Read the model definition and answer for the solid it produces. Units are mm, in the model's axes. Face numbers are marked on the shaded views. A direction names the side the tool comes from. Give positions to 0.01 mm unless a question says otherwise; leave off trailing zeros. Order: outer loops, then holes, each group sorted by start corner. A loop starts at its lowest first (then second) coordinate and runs counter-clockwise, first axis right, second up.
Item 1: Find the intervals of material crossed by line 1 along Y through (x, z) = (-18, 0.9); line 2 along X through (y, z) = (-19.5, 5.5); line 3 along X through (y, z) = (26, 0.55), in increasing order.
Item 2: A cutting plane is placed at D-D (z = 1.9). State how many separate pieces and enclosed holes the cut face has, plus the area to 3 significant figures.
Item 3: Which of the six approach directions +Z, -Z, +X, -X, +Y, -Y give full straight-line access (tool end or side, diameter ignored) to the marked faces 1, 2 and 3?
Item 4: A cutting plane is placed at A-A (y = 21). Write down the section's boundary in (x, z), plus the area to 3 significant figures.
Item 5: Given pin 1 Ø2 at (x, y) = (-4.5, 7) entering from +Z; pin 2 Ø2 at (y, z) = (19.5, 2) entering from +X; pin 3 Ø5 at (x, y) = (7, 24) entering from +Z (3 decimals), each flat-ended and moving along its own axis, determine where each tip first touches the part or whether it passes through.
Item 6: A cutting plane is placed at C-C (x = -5). Write down the section's boundary in (y, z).
Item 7: A cutting plane is placed at B-B (y = 4.5). Write down the section's boundary in (x, z), plus the area to 3 significant figures.
Item 8: The mould has two halves that part along X. Classify the marked faces 4, 5 and 6: +X half, -X half, draft (parallel to the pull), parting line (faces both ways), or undercut.
Autodesk Fusion 360 part; units mm, degrees
sketch "Sketch1" plane through (0, 0, 0) normal (0, 0, 1) x (1, 0, 0)
  circle A0 centre (0, 0) radius 12
  circle A1 centre (0, 0) radius 10
  line L0 (12, 0) -> (0, -12)
  line L1 (-12, 0) -> (0, -12)
  line L2 (-12, 0) -> (0, 12)
  line L3 (0, 12) -> (12, 0)
  line L4 (0, 12) -> (14.1421, 26.1421)
  line L5 (12, 0) -> (26.1421, 14.1421)
  line L6 (26.1421, 14.1421) -> (14.1421, 26.1421)
  line L7 (12, 0) -> (26.1421, -14.1421)
  line L8 (0, -12) -> (14.1421, -26.1421)
  line L9 (14.1421, -26.1421) -> (26.1421, -14.1421)
  line L10 (0, -12) -> (-14.1421, -26.1421)
  line L11 (-12, 0) -> (-26.1421, -14.1421)
  line L12 (-26.1421, -14.1421) -> (-14.1421, -26.1421)
  line L13 (0, 12) -> (-14.1421, 26.1421)
  line L14 (-12, 0) -> (-26.1421, 14.1421)
  line L15 (-26.1421, 14.1421) -> (-14.1421, 26.1421)
  line L16 (16.7761, -9.0966) -> (8.8934, -17.5344)
  line L17 (8.8934, -17.5344) -> (12.2594, -28.5799)
  line L18 (12.2594, -28.5799) -> (23.5081, -31.1876)
  line L19 (23.5081, -31.1876) -> (31.3908, -22.7498)
  line L20 (31.3908, -22.7498) -> (28.0248, -11.7043)
  line L21 (28.0248, -11.7043) -> (16.7761, -9.0966)
  line L22 (-28.0248, -11.7043) -> (-31.3908, -22.7498)
  line L23 (-31.3908, -22.7498) -> (-23.5081, -31.1876)
  line L24 (-23.5081, -31.1876) -> (-12.2594, -28.5799)
  line L25 (-12.2594, -28.5799) -> (-8.8934, -17.5344)
  line L26 (-8.8934, -17.5344) -> (-16.7761, -9.0966)
  line L27 (-16.7761, -9.0966) -> (-28.0248, -11.7043)
  line L28 (-11.7043, 28.0248) -> (-22.7498, 31.3908)
  line L29 (-22.7498, 31.3908) -> (-31.1876, 23.5081)
  line L30 (-31.1876, 23.5081) -> (-28.5799, 12.2594)
  line L31 (-28.5799, 12.2594) -> (-17.5344, 8.8934)
  line L32 (-17.5344, 8.8934) -> (-9.0966, 16.7761)
  line L33 (-9.0966, 16.7761) -> (-11.7043, 28.0248)
  line L34 (9.0966, 16.7761) -> (17.5344, 8.8934)
  line L35 (17.5344, 8.8934) -> (28.5799, 12.2594)
  line L36 (28.5799, 12.2594) -> (31.1876, 23.5081)
  line L37 (31.1876, 23.5081) -> (22.7498, 31.3908)
  line L38 (22.7498, 31.3908) -> (11.7043, 28.0248)
  line L39 (11.7043, 28.0248) -> (9.0966, 16.7761)
  point P0 (20.1421, -20.1421)
  point P1 (-20.1421, -20.1421)
  point P2 (-20.1421, 20.1421)
  point P3 (20.1421, 20.1421)
  dimension "d2" = 20
  dimension "d3" = 20
  dimension "d4" = 20
  dimension "d5" = 20
  dimension "d6" = 20
  dimension "d7" = 20
  dimension "d8" = 20
  dimension "d9" = 20
  dimension "d10" = 10
  dimension "d11" = 10
  dimension "d12" = 10
  dimension "d13" = 10
sketch "Sketch2" plane through (0, 0, 0) normal (0, 0, 1) x (1, 0, 0)
  line L0 (-13.3568, 26.4188) -> (-22.2373, 28.9626)
  line L1 (-22.2373, 28.9626) -> (-28.8805, 22.5437)
  line L2 (-28.8805, 22.5437) -> (-26.6432, 13.5812)
  line L3 (-26.6432, 13.5812) -> (-17.7627, 11.0374)
  line L4 (-17.7627, 11.0374) -> (-11.1195, 17.4563)
  line L5 (-11.1195, 17.4563) -> (-13.3568, 26.4188)
  line L6 (17.5255, 11.1) -> (26.4704, 13.407)
  line L7 (26.4704, 13.407) -> (28.9449, 22.307)
  line L8 (28.9449, 22.307) -> (22.4745, 28.9)
  line L9 (22.4745, 28.9) -> (13.5296, 26.593)
  line L10 (13.5296, 26.593) -> (11.0551, 17.693)
  line L11 (11.0551, 17.693) -> (17.5255, 11.1)
  line L12 (10.8946, -18.4429) -> (14.0988, -27.107)
  line L13 (14.0988, -27.107) -> (23.2042, -28.6641)
  line L14 (23.2042, -28.6641) -> (29.1054, -21.5571)
  line L15 (29.1054, -21.5571) -> (25.9012, -12.893)
  line L16 (25.9012, -12.893) -> (16.7958, -11.3359)
  line L17 (16.7958, -11.3359) -> (10.8946, -18.4429)
  line L18 (-17.6342, -11.0705) -> (-26.5503, -13.4864)
  line L19 (-26.5503, -13.4864) -> (-28.9161, -22.4159)
  line L20 (-28.9161, -22.4159) -> (-22.3658, -28.9295)
  line L21 (-22.3658, -28.9295) -> (-13.4497, -26.5136)
  line L22 (-13.4497, -26.5136) -> (-11.0839, -17.5841)
  line L23 (-11.0839, -17.5841) -> (-17.6342, -11.0705)
  point P0 (-20, 20)
  point P1 (20, 20)
  point P2 (20, -20)
  point P3 (-20, -20)
  dimension "d14" = 8
  dimension "d15" = 8
  dimension "d16" = 8
  dimension "d17" = 8
extrude "Extrude1" add sketch "Sketch2" sketch "Sketch1" along normal blind 6 contours L0 L1 L2 L3 L4 L5 | L6 L7 L8 L9 L10 L11 | L18 L19 L20 L21 L22 L23 of sketch 2 contours L4 L5 L6 L34 L35 L39 | L4 L5 L6 L35 L36 L37 L38 L39 | L7 L8 L9 L17 L18 L19 L20 L21 | L7 L8 L9 L16 L17 L21 | L13 L14 L15 L31 L32 L33 | L13 L14 L15 L28 L29 L30 L31 L33 | L10 L11 L12 L22 L23 L24 L25 L27 | L10 L11 L12 L25 L26 L27 makes body 1 at (-17.3295, 22.7697, 0) makes body 2 at (23.824, 21.2641, 0) makes body 3 at (-16.3926, -19.2729, 0) makes body 4 at (23.8917, -21.0114, 0)
extrude "Extrude2" add sketch "Sketch1" along normal blind 6 separate body contours A0 A1 L3 | A0 A1 L0 | A1 L0 L3 | A0 A1 L2 | A1 L2 L3 | A1 L0 L1 | A0 A1 L1 | A1 L0 | A1 L3 | A1 L1 L2 | A1 L2 | A1 L1 makes body 5
extrude "Extrude3" add sketch "Sketch1" along normal blind 4 contours A0 L7 L8 L16 L17 L21 | A0 L4 L5 L34 L35 L39 | A0 L13 L14 L31 L32 L33 | A0 L10 L11 L25 L26 L27 bodies 5 1 2 3 4
extrude "Extrude4" cut sketch "Sketch2" along normal blind 6 bodies 5
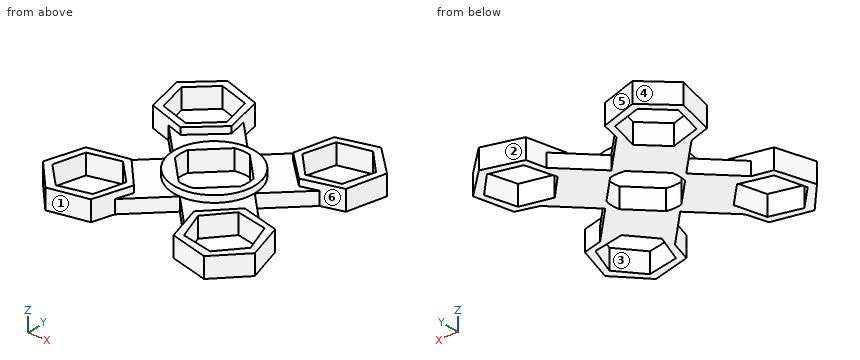
Response values:
1. line 1: y = -29.91 to -27.75, -11.17 to -6, 6 to 11.11, 27.75 to 29.94
1. line 2: x = -30.4 to -28.14, -11.59 to -9.49, 9.49 to 11.29, 28.34 to 30.4
1. line 3: x = -28.52 to -25.3, -13.25 to -11.23, 11.23 to 13.36, 25.32 to 28.52
2. separate pieces: 1
2. enclosed holes: 5
2. area: 1,250 mm2
3. face 1: +Z, -Z, -Y
3. face 2: +Z, -Z, +Y
3. face 3: +Z, -Z
4. outline: (-30.61, 0) - (-28.5, 0) - (-28.5, 6) - (-30.61, 6) - close; (-12, 0) - (-9, 0) - (-9, 4) - (-10.08, 4) - (-10.08, 6) - (-12, 6) - close; (9, 0) - (11.97, 0) - (11.97, 6) - (10.08, 6) - (10.08, 4) - (9, 4) - close; (28.58, 0) - (30.61, 0) - (30.61, 6) - (28.58, 6) - close
4. area: 56.4 mm2
5. pin 1: stops at z = 6
5. pin 2: stops at x = 30.49
5. pin 3: passes through
6. outline: (-17, 0) - (-7, 0) - (-7, 6) - (-10.91, 6) - (-10.91, 4) - (-17, 4) - close; (7, 0) - (17, 0) - (17, 4) - (10.91, 4) - (10.91, 6) - (7, 6) - close
7. outline: (-16.5, 0) - (-7.5, 0) - (-7.5, 6) - (-11.12, 6) - (-11.12, 4) - (-16.5, 4) - close; (7.5, 0) - (16.5, 0) - (16.5, 4) - (11.12, 4) - (11.12, 6) - (7.5, 6) - close
7. area: 86.5 mm2
8. face 4: -X half
8. face 5: undercut
8. face 6: +X half
